```python
from build123d import *

# Parameters (mm, degrees)
F0_R     = 39.244095
F1_DEPTH = 15.24
F3_R     = 39.244095
F3_R_2   = 3.81
F3_R_3   = 4.493743
F4_DEPTH = 12.7
F5_R     = 5.08


with BuildPart() as f1:
    # F0 (on Top) → F1 (new body)
    with BuildSketch(Plane.XY):
        Circle(F0_R)
    extrude(amount=F1_DEPTH)

    # F3 (on face) → F4 (join)
    with BuildSketch(Plane.XY.offset(15.24)):
        Circle(F3_R)
        with Locations((0, -25.4)):
            Circle(F3_R_2, mode=Mode.SUBTRACT)
        with Locations((-25.4, 0)):
            Circle(F3_R_2, mode=Mode.SUBTRACT)
        with Locations((25.4, 0)):
            Circle(F3_R_2, mode=Mode.SUBTRACT)
        with Locations((0, 29.893743)):
            Circle(F3_R_3, mode=Mode.SUBTRACT)
    extrude(amount=F4_DEPTH)

    # F5
    f5_edges = [f1.edges().sort_by_distance(p)[0] for p in [
        (-39.244095, 0, 0),
    ]]
    fillet(f5_edges, radius=F5_R)


solid = f1.part
```
Verification items for the finished model (mm, model axes). A direction names the side the tool comes from. Coordinates: 2 decimals unless noted, no trailing zeros. Loops run counter-clockwise (first coordinate to the right, second up) from the corner with the lowest first, then second, coordinate; pieces in that order, holes last. Notation, with made-up numbers: (65.5, -7.75) -> (89.5, -7.75) arc R19 cw to (89.5, 3.25) -> close; hole circle Ø1 at (-4, -26.75). An arc over 180 degrees is marked (long way). Answer in a Markdown table with one row per item. Add a question column.
1. Section check C-C, the plane z = 13.25. Enter the section's corners in (x, y).
2. Section check A-A, the plane x = 0. Enter the section's corners in (y, z), then the cut area to 3 significant figures.
3. Section check B-B, the plane z = 22.5. Enter the section's corners in (x, y).
4. Material ranges on probe 1 along Y at (x, z) = (0, 18); probe 2 along X at (y, z) = (1, 20); probe 3 along Z at (x, y) = (0, 33), recorded low to high. Write a range as [from, to].
5. Depth check by flat-ended pin: P1, Ø8, axis at y = -6, z = 15, coming from the +X side; P2, Ø1.5, axis at y = -23.5, z = 3.5, coming from the -X side; P3, Ø2.5, axis at x = -26.5, y = 1, coming from the +Z side; P4, Ø4.5, axis at x = -25.4, y = 0, coming from the -Z side. Enter the tip coordinate at first touch or a pass-through.
6. Access from +Z, -Z, +X, -X, +Y, -Y to the whole of each face (thin tool, end or side, straight path). Record for faces 1 (the face through (28.92, -1.46, 21.5)), 2 (the face through (-1, 1, 27.94)).
7. Draft check along X on faces 3 (the face through (0, 0, 0)), 4 (the face through (0, -25, 15.24)), 5 (the face through (-8.51, -38.31, 16.35)). Enter one of: +X half, -X half, draft (parallel to the pull), parting line (faces both ways), or undercut.
Derived:
| question | item | result |
|---|---|---|
| 1 | outline | circle Ø78.49 at (0, 0) |
| 2 | outline | (-39.24, 5.08) arc R5.08 ccw to (-34.16, 0) -> (34.16, 0) arc R5.08 ccw to (39.24, 5.08) -> (39.24, 27.94) -> (34.39, 27.94) -> (34.39, 15.24) -> (25.4, 15.24) -> (25.4, 27.94) -> (-21.59, 27.94) -> (-21.59, 15.24) -> (-29.21, 15.24) -> (-29.21, 27.94) -> (-39.24, 27.94) -> close |
| 2 | area | 1,970 mm² |
| 3 | outline | circle Ø78.49 at (0, 0); hole circle Ø7.62 at (-25.4, 0); hole circle Ø8.99 at (0, 29.89); hole circle Ø7.62 at (0, -25.4); hole circle Ø7.62 at (25.4, 0) |
| 4 | probe 1 | y = [-39.24, -29.21], [-21.59, 25.4], [34.39, 39.24] |
| 4 | probe 2 | x = [-39.23, -29.08], [-21.72, 21.72], [29.08, 39.23] |
| 4 | probe 3 | z = [0, 15.24] |
| 5 | P1 | stops at x = 39.19 |
| 5 | P2 | stops at x = -31.73 |
| 5 | P3 | stops at z = 15.24 |
| 5 | P4 | stops at z = 0 |
| 6 | face 1 | +Z |
| 6 | face 2 | +Z, +X, -X, +Y, -Y |
| 7 | face 3 | draft |
| 7 | face 4 | undercut |
| 7 | face 5 | parting line |
